Source: CAD feature listing. Evaluate the final solid. Frame: model axes, mm. A direction names the side the tool comes from. Coordinates: 2 decimals unless noted, no trailing zeros. Order: outer loops, then holes, each group sorted by start corner. A loop starts at its lowest first (then second) coordinate and runs counter-clockwise, first axis right, second up. Notation, with made-up numbers: (21, 2.5) - (49, 2.5) arc R28 ccw to (49, 34.5) - close; hole circle Ø3 at (-38.5, 5). An arc over 180 degrees is marked (long way). One line per question, with ' | ' between items.
from build123d import *

# Parameters (mm, degrees)
SKETCH1_R                = 2.5
BOSS_EXTRUDE1_DEPTH      = 20
SKETCH24_W               = 8.1
SKETCH24_H               = 25
SKETCH24_W_2             = 3.1
CUT_EXTRUDE14_DEPTH      = 9
CUT_EXTRUDE14_DEPTH_BACK = 9
SKETCH25_R               = 1
CUT_EXTRUDE15_DEPTH      = 4
CUT_EXTRUDE15_DEPTH_BACK = 14
SKETCH31_W               = 4
SKETCH31_H               = 25
CUT_EXTRUDE17_DEPTH      = 4
CUT_EXTRUDE17_DEPTH_BACK = 14
BOSS_EXTRUDE5_START      = -20
BOSS_EXTRUDE5_DEPTH      = 20
SKETCH32_R               = 2.5
BOSS_EXTRUDE6_DEPTH      = 2


with BuildPart() as part:
    # Sketch1 → Boss-Extrude1 (new body)
    with BuildSketch(Plane(origin=(0, 0, 0), x_dir=(0, 0, -1), z_dir=(1, 0, 0))):
        with BuildLine():
            Line((-5, 22.270117322), (-5, 7.475642404))
            ThreePointArc((-5, 7.475642404), (-3.411481861, -24.340079768), (-7.786398999, -55.893584601))
            ThreePointArc((-7.786398999, -55.893584601), (0, -65.729882678), (7.786398999, -55.893584601))
            ThreePointArc((7.786398999, -55.893584601), (3.411481861, -24.340079768), (5, 7.475642404))
            Line((5, 7.475642404), (5, 22.270117322))
            ThreePointArc((5, 22.270117322), (0, 27.270117322), (-5, 22.270117322))
        make_face()
        with Locations((0, -57.729882678)):
            Circle(SKETCH1_R, mode=Mode.SUBTRACT)
        with BuildLine():
            Line((1.5, 12.475642404), (1.5, 17.270117322))
            ThreePointArc((1.5, 17.270117322), (0, 18.770117322), (-1.5, 17.270117322))
            Line((-1.5, 17.270117322), (-1.5, 12.475642404))
            ThreePointArc((-1.5, 12.475642404), (0, 10.975642404), (1.5, 12.475642404))
        make_face(mode=Mode.SUBTRACT)
    extrude(amount=BOSS_EXTRUDE1_DEPTH)

    # Sketch24 → Cut-Extrude14 (cut, two sides)
    with BuildSketch(Plane.XY) as cut_extrude14_sk:
        with Locations((4.05, -53.229882678)):
            Rectangle(SKETCH24_W, SKETCH24_H)
        with Locations((18.45, -53.229882678)):
            Rectangle(SKETCH24_W_2, SKETCH24_H)
    extrude(amount=CUT_EXTRUDE14_DEPTH, mode=Mode.SUBTRACT)
    extrude(cut_extrude14_sk.sketch, amount=-CUT_EXTRUDE14_DEPTH_BACK, mode=Mode.SUBTRACT)

    # Sketch25 → Cut-Extrude15 (cut, two sides)
    with BuildSketch(Plane(origin=(0, 0, -5), x_dir=(-1, 0, 0), z_dir=(0, 0, -1))) as cut_extrude15_sk:
        with Locations((-17, 9.225642404)):
            Circle(SKETCH25_R)
        with Locations((-17, 20.520117322)):
            Circle(SKETCH25_R)
        with Locations((-3, 9.225642404)):
            Circle(SKETCH25_R)
        with Locations((-3, 20.520117322)):
            Circle(SKETCH25_R)
    extrude(amount=CUT_EXTRUDE15_DEPTH, mode=Mode.SUBTRACT)
    extrude(cut_extrude15_sk.sketch, amount=-CUT_EXTRUDE15_DEPTH_BACK, mode=Mode.SUBTRACT)

    # Sketch31 → Cut-Extrude17 (cut, two sides)
    with BuildSketch(Plane.XY.offset(5)) as cut_extrude17_sk:
        with Locations((10.1, -53.229882678)):
            Rectangle(SKETCH31_W, SKETCH31_H)
    extrude(amount=CUT_EXTRUDE17_DEPTH, mode=Mode.SUBTRACT)
    extrude(cut_extrude17_sk.sketch, amount=-CUT_EXTRUDE17_DEPTH_BACK, mode=Mode.SUBTRACT)

    # Sketch26 → Boss-Extrude5 (add)
    with BuildSketch(Plane(origin=(20, 0, 0), x_dir=(0, 0, -1), z_dir=(1, 0, 0)).offset(BOSS_EXTRUDE5_START)):
        with BuildLine():
            Line((-4.929780951, -40.729882678), (4.929780951, -40.729882678))
            ThreePointArc((4.929780951, -40.729882678), (0, -43.50073532), (-4.929780951, -40.729882678))
        make_face()
    extrude(amount=BOSS_EXTRUDE5_DEPTH)

    # Sketch32 → Boss-Extrude6 (add)
    with BuildSketch(Plane.ZY.offset(-12.1)):
        with BuildLine():
            Line((-2.5, -53.227383372), (-2.5, -42.931107555))
            Line((-2.5, -42.931107555), (2.5, -42.931107555))
            Line((2.5, -42.931107555), (2.5, -53.227383372))
            ThreePointArc((2.5, -53.227383372), (0, -62.879882678), (-2.5, -53.227383372))
        make_face()
        with Locations((0, -57.729882678)):
            Circle(SKETCH32_R, mode=Mode.SUBTRACT)
    extrude(amount=BOSS_EXTRUDE6_DEPTH)


solid = part.part
(1) Cut plane A-A (x = 3). Return the cut outline in (y, z), and give its area (3 significant figures).
Taken from the geometry:
outline: (-40.73, -4.93) arc R170 cw to (7.48, -5) - (8.23, -5) - (8.23, 5) - (7.48, 5) arc R170 cw to (-40.73, 4.93) arc R5.77 ccw to start; (10.23, -5) - (19.52, -5) - (19.52, 5) - (10.23, 5) - close; (21.52, -5) - (22.27, -5) arc R5 ccw to (22.27, 5) - (21.52, 5) - close; hole (12.48, -1.5) - (17.27, -1.5) arc R1.5 ccw to (17.27, 1.5) - (12.48, 1.5) arc R1.5 ccw to start | area: 513 mm²
(2) Cut plane C-C (y = 4.5). Return the cut outline in (x, z).
Taken from the geometry:
outline: (0, -4.6) - (20, -4.6) - (20, 4.6) - (0, 4.6) - close
(3) Set-up query: faces 4 (the flat face through (10, 15, -5)), 5 (the cylindrical face through (9.86, 10.976, 0.033)), 6 (the flat face through (10, 15, 5)). Return all of +Z, -Z, +X, -X, +Y, -Y with unobstructed straight access to the full face (end or side cutting, diameter ignored); none if empty.
Taken from the geometry:
face 4: -Z, +X, -X, +Y | face 5: +X, -X | face 6: +Z, +X, -X, +Y
(4) Material intervals for L1, parallel to Y at x = 15.75, z = 0; L2, parallel to Y at x = 17, z = 1; L3, parallel to Z at x = 5.25, y = -15.5, sorted ascending. Write a range as from..to.
Taken from the geometry:
L1: y = -65.73..-60.23, -55.23..10.98, 18.77..27.27 | L2: y = -43.41..8.23, 10.23..11.36, 18.39..19.52, 21.52..27.17 | L3: z = -3.25..3.25
(5) Pin query (flat end, axial travel): P1, Ø4.5, axis at x = 14, y = 18, coming from the -Z side; P2, Ø4.5, axis at x = 8.5, y = 15.5, coming from the +Z side; P3, Ø1, axis at y = -7.5, z = -2.5, coming from the -X side; P4, Ø3, axis at y = -50, z = 0, coming from the -X side. Return the tip coordinate at first contact, or that it passes through.
Taken from the geometry:
P1: stops at z = -5 | P2: stops at z = 5 | P3: stops at x = 0 | P4: stops at x = 10.1
(6) Cut plane B-B (z = 0). Return the cut outline in (x, y), and give its area (3 significant figures).
Taken from the geometry:
outline: (0, -43.5) - (10.1, -43.5) - (10.1, -55.23) - (16.9, -55.23) - (16.9, -43.5) - (20, -43.5) - (20, 10.98) - (0, 10.98) - close; (0, 18.77) - (20, 18.77) - (20, 27.27) - (0, 27.27) - close; (10.1, -62.88) - (12.1, -62.88) - (12.1, -65.73) - (16.9, -65.73) - (16.9, -60.23) - (10.1, -60.23) - close; hole circle Ø2 at (3, 9.23); hole circle Ø2 at (3, 20.52); hole circle Ø2 at (17, 9.23); hole circle Ø2 at (17, 20.52) | area: 1,360 mm²
(7) Pull-direction query (Y, two-part tool) for faces 1 (the flat face through (10.1, -53, 0)), 2 (the flat face through (10, 15, 1.5)), 3 (the cylindrical face through (18.4, -43.5, -0.1)); classes: pulls with the +Y half, pulls with the -Y half, needs draft (parallel to the pull), parting line crosses it, or undercut.
Taken from the geometry:
face 1: needs draft | face 2: undercut | face 3: pulls with the -Y half
